```python
from build123d import *

# Parameters (mm, degrees)
SZKIC1_W                    = 11
SZKIC1_H                    = 145
DODANIE_WYCI_GNI_CIE1_DEPTH = 1.9
SZKIC3_W                    = 11
SZKIC3_H                    = 16
WYTNIJ_WYCI_GNI_CIE1_DEPTH  = 0.9
SFAZOWANIE1_SIZE            = 1
SZKIC2_W                    = 11
SZKIC2_H                    = 6
DODANIE_WYCI_GNI_CIE2_DEPTH = 6
ZAOKR_GLENIE1_R             = 1


with BuildPart() as part:
    # Szkic1 → Dodanie-wyciągnięcie1 (new body)
    with BuildSketch(Plane(origin=(0, 0, 0), x_dir=(1, 0, 0), z_dir=(0, 1, 0))):
        Rectangle(SZKIC1_W, SZKIC1_H)
    extrude(amount=DODANIE_WYCI_GNI_CIE1_DEPTH)

    # Szkic3 → Wytnij-wyciągnięcie1 (cut)
    with BuildSketch(Plane(origin=(0, 1.9, 0), x_dir=(1, 0, 0), z_dir=(0, 1, 0))):
        with Locations((0, 64.5)):
            Rectangle(SZKIC3_W, SZKIC3_H)
    extrude(amount=-WYTNIJ_WYCI_GNI_CIE1_DEPTH, mode=Mode.SUBTRACT)

    # Sfazowanie1
    # the kernel refuses this chamfer: 1 mm, written as the material it takes off along each edge
    with BuildSketch(Plane(origin=(-8.071682988, 1.9, -56.5), x_dir=(0, 0.0274958766105862, 0.9996219169112968), z_dir=(1, 0, 0))) as sfazowanie1_piece_1_section:
        Polygon((SFAZOWANIE1_SIZE * 0.999621916911, SFAZOWANIE1_SIZE * 0.0274958766106), (-SFAZOWANIE1_SIZE * 0.0274958766106, SFAZOWANIE1_SIZE * 0.999621916911), (0, 0), align=None)
    sfazowanie1_piece_1 = extrude(amount=16.143365976, mode=Mode.PRIVATE)
    sfazowanie1_piece_1 = split(sfazowanie1_piece_1, bisect_by=Plane(origin=(0, 1, -56.164099253), z_dir=(0, 1, 0)), keep=Keep.TOP, mode=Mode.PRIVATE)
    add(sfazowanie1_piece_1, mode=Mode.SUBTRACT)
    with BuildSketch(Plane(origin=(8.071682988, 1, -72.5), x_dir=(0, -0.999621916911297, -0.02749587661058218), z_dir=(-1, 0, 0))) as sfazowanie1_piece_2:
        Polygon((SFAZOWANIE1_SIZE * 0.999621916911, SFAZOWANIE1_SIZE * 0.0274958766106), (-SFAZOWANIE1_SIZE * 0.0274958766106, SFAZOWANIE1_SIZE * 0.999621916911), (0, 0), align=None)
    extrude(amount=16.143365976, mode=Mode.SUBTRACT)

    # Szkic2 → Dodanie-wyciągnięcie2 (add)
    with BuildSketch(Plane(origin=(0, 1.9, 0), x_dir=(1, 0, 0), z_dir=(0, 1, 0))):
        with Locations((0, -64.5)):
            Rectangle(SZKIC2_W, SZKIC2_H)
    extrude(amount=DODANIE_WYCI_GNI_CIE2_DEPTH)

    # Zaokrąglenie1
    zaokr_glenie1_edges = [part.edges().sort_by_distance(p)[0] for p in [
        (5.5, 0.5, -72),
        (-5.5, 0.5, -72),
        (0, 1.9, 67.5),
        (0, 1.9, 61.5),
        (0, 7.9, 67.5),
        (0, 7.9, 61.5),
        (5.5, 0.95, 72.5),
        (-5.5, 0.95, 72.5),
    ]]
    fillet(zaokr_glenie1_edges, radius=ZAOKR_GLENIE1_R)


solid = part.part
```
Input: part model. Units: mm. Frame: model coordinates. A direction names the side the tool comes from. Coordinates: 2 decimals unless noted, no trailing zeros. Order: outer loops, then holes, each group sorted by start corner. A loop starts at its lowest first (then second) coordinate and runs counter-clockwise, first axis right, second up. Notation, with made-up numbers: (-29.75, -12) - (-11.75, -12) arc R26 cw to (-11.75, 17) - close; hole circle Ø11 at (87, 42). An arc over 180 degrees is marked (long way). Put each result on its own line as item: value.
1. Reachability of faces 1 (the face through (0, 1, -64)), 2 (the face through (0, 7.9, 64)), 3 (the face through (0, 5, 67.5)) from +Z, -Z, +X, -X, +Y, -Y: full face, straight path, thin tool, end or side. Return the list, or none.
Report:
face 1: -Z, +X, -X, +Y
face 2: +Z, -Z, +X, -X, +Y
face 3: +Z, +X, -X, +Y
2. Cut plane A-A on x = -3. Return the cut outline in (y, z), then the cut area to 3 significant figures.
Report:
outline: (0, -72.5) - (1, -71.5) - (1, -56.4) - (1.9, -55.5) - (1.9, 60.5) arc R1 cw to (2.9, 61.5) - (6.9, 61.5) arc R1 ccw to (7.9, 62.5) - (7.9, 66.5) arc R1 ccw to (6.9, 67.5) - (2.9, 67.5) arc R1 cw to (1.9, 68.5) - (1.9, 72.5) - (0, 72.5) - close
area: 296 mm2
3. Line query: line 1 along Y through (x, z) = (-1.75, -61); line 2 along Y through (x, z) = (3.75, -27); line 3 along Z through (x, y) = (3.75, 6.75). Output: solid intervals per line, ascending.
Report:
line 1: y = 0 to 1
line 2: y = 0 to 1.9
line 3: z = 61.5 to 67.5
4. Contact query for flat-ended pins moving along their axis: pin 1 Ø1.5 at (x, y) = (-4, 4.5) entering from +Z; pin 2 Ø3.5 at (x, z) = (1.5, -10.5) entering from +Y; pin 3 Ø3 at (x, y) = (-3, 6) entering from -Z; pin 4 Ø1.5 at (y, z) = (2, 45) entering from -X. Output: stop coordinate, or through.
Report:
pin 1: stops at z = 67.5
pin 2: stops at y = 1.9
pin 3: stops at z = 61.5
pin 4: stops at x = -5.5
5. Cut plane C-C on z = 12.5. Return the cut outline in (x, y), then the cut area to 3 significant figures.
Report:
outline: (-5.5, 0) - (5.5, 0) - (5.5, 1.9) - (-5.5, 1.9) - close
area: 20.9 mm2
6. Cut plane B-B on y = 5.5. Return the cut outline in (x, z), then the cut area to 3 significant figures.
Report:
outline: (-5.5, 61.5) - (5.5, 61.5) - (5.5, 67.5) - (-5.5, 67.5) - close
area: 66.0 mm2
